Geometry check sheet. Reference: the model listing, model coordinates, mm. Face numbers are marked on the shaded views. A direction names the side the tool comes from. Round coordinates to 2 decimals unless told otherwise and drop trailing zeros. Order: outer loops, then holes, each group sorted by start corner. A loop starts at its lowest first (then second) coordinate and runs counter-clockwise, first axis right, second up. Notation, with made-up numbers: M 39.5,77.5 L 96.5,77.5 A20 ccw 96.5,108.5 Z; hole C -9.75,42 d5. An arc over 180 degrees is marked long. Return JSON: item names as keys, results as strings. Group by question number.
```python
from build123d import *

# Parameters (mm, degrees)
SKETCH1_R           = 2.25
SKETCH1_R_2         = 0.75
BOSS_EXTRUDE1_DEPTH = 4.7
CUT_EXTRUDE1_DEPTH  = 5.7
CHAMFER1_SIZE       = 1


with BuildPart() as part:
    # Sketch1 → Boss-Extrude1 (new body)
    with BuildSketch(Plane.XY):
        with BuildLine():
            Line((2, 0), (18, 0))
            ThreePointArc((18, 0), (19.414213562, 0.585786438), (20, 2))
            Line((20, 2), (20, 28))
            ThreePointArc((20, 28), (19.414213562, 29.414213562), (18, 30))
            Line((18, 30), (2, 30))
            ThreePointArc((2, 30), (0.585786438, 29.414213562), (0, 28))
            Line((0, 28), (0, 2))
            ThreePointArc((0, 2), (0.585786438, 0.585786438), (2, 0))
        make_face()
        with Locations((10, 23)):
            Circle(SKETCH1_R, mode=Mode.SUBTRACT)
        with Locations((6.85, 4.8)):
            Circle(SKETCH1_R_2, mode=Mode.SUBTRACT)
        with Locations((13.15, 4.8)):
            Circle(SKETCH1_R_2, mode=Mode.SUBTRACT)
    extrude(amount=BOSS_EXTRUDE1_DEPTH)

    # Sketch2 → Cut-Extrude1 (cut, through all)
    with BuildSketch(Plane.XY.offset(4.7)):
        with BuildLine():
            Line((20, 16.5), (10, 16.5))
            ThreePointArc((10, 16.5), (7.5, 14), (10, 11.5))
            Line((10, 11.5), (20, 11.5))
            Line((20, 11.5), (20, 16.5))
        make_face()
    extrude(amount=-CUT_EXTRUDE1_DEPTH, mode=Mode.SUBTRACT)

    # Chamfer1
    chamfer1_edges = [part.edges().sort_by_distance(p)[0] for p in [
        (15, 11.5, 0),
        (7.5, 14, 0),
        (15, 16.5, 0),
        (15, 16.5, 4.7),
        (7.5, 14, 4.7),
        (15, 11.5, 4.7),
    ]]
    chamfer(chamfer1_edges, length=CHAMFER1_SIZE)


solid = part.part
```
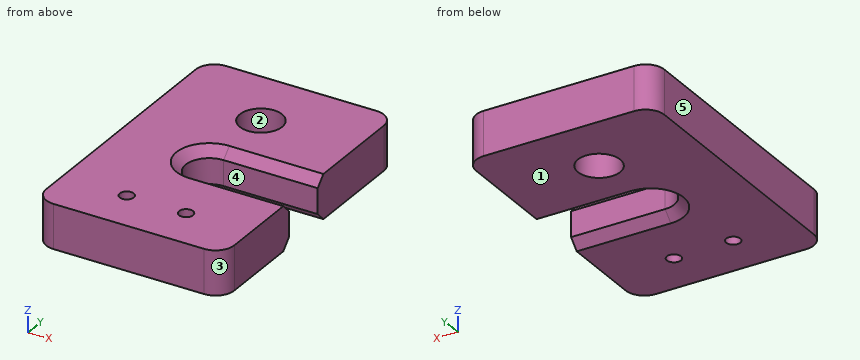
Q1. Material ranges on line 1 along Y through (x, z) = (13.15, 1.55); line 2 along Y through (x, z) = (6.85, 3.4); line 3 along Y through (x, z) = (15.25, 1.1), recorded low to high.
Q2. Depth check by flat-ended pin: pin 1 Ø2 at (x, z) = (8, 3) entering from -Y; pin 2 Ø2.5 at (x, y) = (10, 23) entering from +Z. Enter the tip coordinate at first touch or a pass-through.
Q3. Set-up check for the marked faces 4 and 5: record each of +Z, -Z, +X, -X, +Y, -Y from which the full face is reachable in a straight line by a thin tool's end or side.
Q4. Release check for a two-part mould opening along X. For the marked faces 1, 2 and 3 record: +X half, -X half, draft (parallel to the pull), parting line (faces both ways), or undercut.
Q5. Section check A-A on y = 23. Record the cut outline in (x, z), plus the area to 4 significant figures.
Q6. Section check C-C on z = 4.4. Record the cut outline in (x, y).
Q7. Section check B-B on y = 4.8. Record the cut outline in (x, z).
Q8. Section check D-D on x = 13.15. Record the cut outline in (y, z).
Geometry check:
{
 "1": {"line 1": "y = 0 to 4.05, 5.55 to 11.5, 16.5 to 30", "line 2": "y = 0 to 4.05, 5.55 to 30", "line 3": "y = 0 to 11.5, 16.5 to 30"},
 "2": {"pin 1": "stops at y = 0", "pin 2": "passes through"},
 "3": {"face 4": "+Z, -Z, +X", "face 5": "+Z, -Z, -X, +Y, -Y"},
 "4": {"face 1": "draft", "face 2": "undercut", "face 3": "+X half"},
 "5": {"outline": "M 0,0 L 7.75,0 L 7.75,4.7 L 0,4.7 Z; M 12.25,0 L 20,0 L 20,4.7 L 12.25,4.7 Z", "area": "72.85 mm^2"},
 "6": {"outline": "M 0,2 A2 ccw 2,0 L 18,0 A2 ccw 20,2 L 20,10.8 L 10,10.8 A3.2 cw 10,17.2 L 20,17.2 L 20,28 A2 ccw 18,30 L 2,30 A2 ccw 0,28 Z; hole C 6.85,4.8 d1.5; hole C 10,23 d4.5; hole C 13.15,4.8 d1.5"},
 "7": {"outline": "M 0,0 L 6.1,0 L 6.1,4.7 L 0,4.7 Z; M 7.6,0 L 12.4,0 L 12.4,4.7 L 7.6,4.7 Z; M 13.9,0 L 20,0 L 20,4.7 L 13.9,4.7 Z"},
 "8": {"outline": "M 0,0 L 4.05,0 L 4.05,4.7 L 0,4.7 Z; M 5.55,0 L 10.5,0 L 11.5,1 L 11.5,3.7 L 10.5,4.7 L 5.55,4.7 Z; M 16.5,1 L 17.5,0 L 30,0 L 30,4.7 L 17.5,4.7 L 16.5,3.7 Z"}
}
